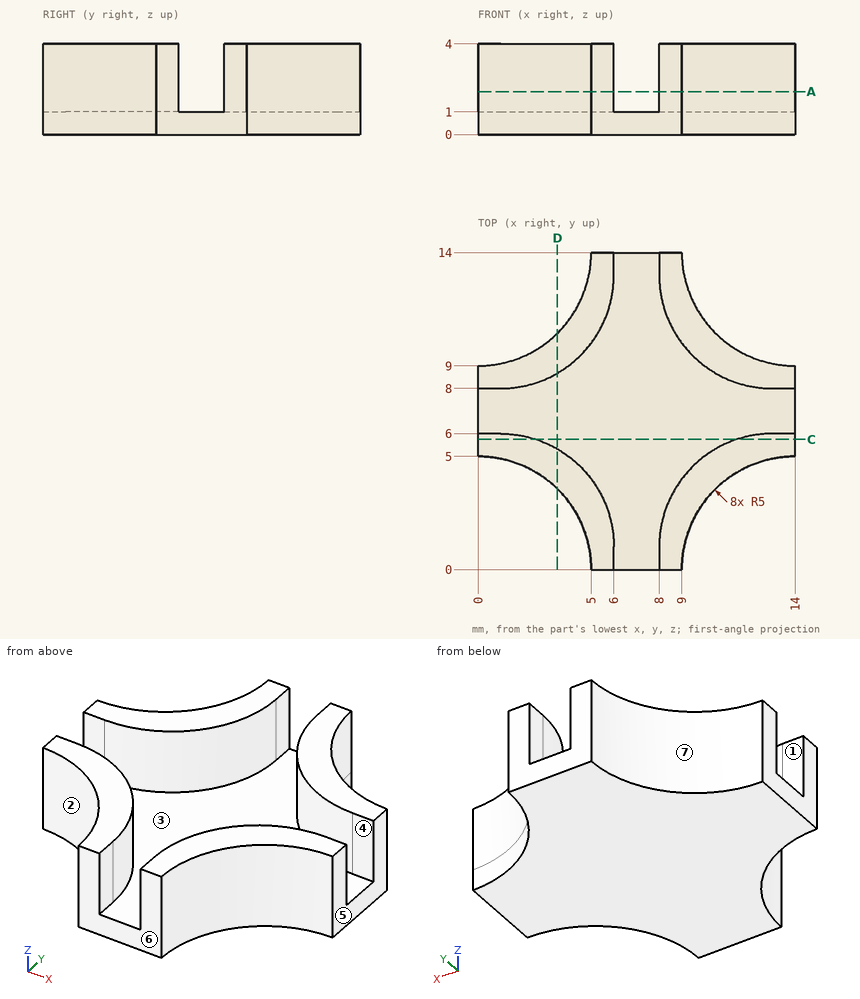
Geometry: see drawing. Coordinates: mm, zero at the bounding-box minimum. A direction names the side the tool comes from. Coordinates: 2 decimals unless noted, no trailing zeros. Loops run counter-clockwise (first coordinate to the right, second up) from the corner with the lowest first, then second, coordinate; pieces in that order, holes last.
(1) First-contact query: pin 1 Ø1.1 at (y, z) = (13.5, 2) entering from +X; pin 2 Ø0.5 at (x, z) = (13.5, 2.5) entering from +Y; pin 3 Ø0.5 at (x, z) = (0.5, 2.5) entering from -Y; pin 4 Ø1 at (x, y) = (10.5, 2.5) entering from +Z. Flat tips, straight axial feed; report the tip coordinate or a pass-through.
(2) Section D-D on x = 3.5. Return the cut outline in (y, z), then the cut area to 3 significant figures.
(3) Section C-C on y = 5.75. Return the cut outline in (x, z).
(4) Material intervals for probe 1 along X at (y, z) = (9.75, 3.7); probe 2 along Z at (x, y) = (6.5, 9); probe 3 along X at (y, z) = (13.75, 1.2), sorted ascending.
(5) Pull-direction query (Y, two-part tool) for the marked faces 4, 5, 6 and 7; classes: released by +Y, released by -Y, zero draft, split by the parting line, or undercut.
(6) Set-up query: the marked faces 1, 2 and 3. Return all of +Z, -Z, +X, -X, +Y, -Y with unobstructed straight access to the full face (end or side cutting, diameter ignored); none if empty.
(7) Section A-A on z = 1.9. Count the separate pieces of the cut face and the enclosed holes in it, then the cut area to 3 significant figures.
Data:
1. pin 1: stops at x = 9.11
1. pin 2: stops at y = 9.06
1. pin 3: stops at y = 4.94
1. pin 4: passes through
2. outline: (3.57, 0) - (10.43, 0) - (10.43, 4) - (8.67, 4) - (8.67, 1) - (5.33, 1) - (5.33, 4) - (3.57, 4) - close
2. area: 17.4 mm2
3. outline: (0, 0) - (14, 0) - (14, 4) - (11.44, 4) - (11.44, 1) - (2.56, 1) - (2.56, 4) - (0, 4) - close
4. probe 1: x = 2.63 to 4.8, 9.2 to 11.37
4. probe 2: z = 0 to 1
4. probe 3: x = 4.99 to 6, 8 to 9.01
5. face 4: undercut
5. face 5: zero draft
5. face 6: released by -Y
5. face 7: released by +Y
6. face 1: +Z, +X, -X
6. face 2: +Z, -Z, -X, -Y
6. face 3: +Z
7. separate pieces: 4
7. enclosed holes: 0
7. area: 44.0 mm2
